For this review, take the finished solid that the model builds, in its own axes (mm). Round coordinates to 2 decimals unless told otherwise and drop trailing zeros. Loops run counter-clockwise (first coordinate to the right, second up) from the corner with the lowest first, then second, coordinate; pieces in that order, holes last. Notation, with made-up numbers: (58.25, 20) -> (86.25, 20) arc R12 ccw to (86.25, 40) -> close; hole circle Ø1 at (57.25, 26.5). An arc over 180 degrees is marked (long way). One line per question, with ' | ' between items. Start each with the question number.
1. Draft analysis for pull direction Y (two halves, no side actions). For faces 1 (the face through (0, 23, -208)), 2 (the face through (3.131, -25.395, -190.081)), 3 (the face through (3.131, 25.395, -190.919)), state which applies: pulls with the +Y half, pulls with the -Y half, needs draft (parallel to the pull), parting line crosses it, or undercut.
2. Consider section A-A (y = 76.2). Write out the cut boundary in (x, z), and give its area (3 significant figures).
3. Consider section C-C (x = 3.75). Count the separate pieces of the cut face and the enclosed holes in it, and give its area (3 significant figures).
4. Wall thickness on line 1 along Z through (x, y) = (5.25, -68.5); line 2 along Z through (x, y) = (1, 20); line 3 along Y through (x, z) = (5.25, -114): over which ranges is each line inside the solid? List them lowest first.
5. Consider section B-B (z = -194). Write out the cut boundary in (x, y).
```python
from build123d import *

# Parameters (mm, degrees)
BOSS_EXTRUDE1_DEPTH = 6.35
SKETCH2_R           = 1.7272
SKETCH2_R_2         = 1.3890625
SKETCH2_R_3         = 1.984375
CUT_EXTRUDE1_DEPTH  = 7.35


with BuildPart() as part:
    # Sketch1 → Boss-Extrude1 (new body)
    with BuildSketch(Plane(origin=(0, 0, 0), x_dir=(0, 0, -1), z_dir=(1, 0, 0))):
        Polygon((146.05, 95.25), (158.75, 95.25), (552.45, 95.25), (552.45, -95.25), (158.75, -95.25), (146.05, -95.25), (-146.05, -95.25), (-146.05, 95.25), align=None)
    extrude(amount=BOSS_EXTRUDE1_DEPTH)

    # Sketch2 → Cut-Extrude1 (cut, through all)
    with BuildSketch(Plane.ZY):
        with Locations((113.660651072, 53.713174026)):
            Circle(SKETCH2_R)
        with Locations((75.560651072, 53.713174026)):
            Circle(SKETCH2_R)
        with Locations((37.460651072, 53.713174026)):
            Circle(SKETCH2_R)
        with Locations((-0.639348928, 53.713174026)):
            Circle(SKETCH2_R)
        with Locations((-38.739348928, 53.713174026)):
            Circle(SKETCH2_R)
        with Locations((-76.839348928, 53.713174026)):
            Circle(SKETCH2_R)
        with Locations((-114.939348928, 53.713174026)):
            Circle(SKETCH2_R)
        with Locations((-114.939348928, 2.913174026)):
            Circle(SKETCH2_R)
        with Locations((-76.839348928, 2.913174026)):
            Circle(SKETCH2_R)
        with Locations((-38.739348928, 2.913174026)):
            Circle(SKETCH2_R)
        with Locations((-0.639348928, 2.913174026)):
            Circle(SKETCH2_R)
        with Locations((37.460651072, 2.913174026)):
            Circle(SKETCH2_R)
        with Locations((75.560651072, 2.913174026)):
            Circle(SKETCH2_R)
        with Locations((113.660651072, 2.913174026)):
            Circle(SKETCH2_R)
        with Locations((92.336825974, -67.314348928)):
            Circle(SKETCH2_R)
        with Locations((41.536825974, -67.314348928)):
            Circle(SKETCH2_R)
        with Locations((-47.363174026, -67.314348928)):
            Circle(SKETCH2_R)
        with Locations((-98.163174026, -67.314348928)):
            Circle(SKETCH2_R)
        with Locations((-227.452489037, 52.197)):
            Circle(SKETCH2_R)
        with Locations((-227.452489037, -52.197)):
            Circle(SKETCH2_R)
        with Locations((-409.722889037, -52.197)):
            Circle(SKETCH2_R)
        with Locations((-409.722889037, 52.197)):
            Circle(SKETCH2_R)
        with Locations((-522.859, -17.782353467)):
            Circle(SKETCH2_R_2)
        with Locations((-479.806, -17.78)):
            Circle(SKETCH2_R_2)
        with Locations((-479.806, -65.532)):
            Circle(SKETCH2_R_2)
        with Locations((-522.859, -65.532)):
            Circle(SKETCH2_R_2)
        with Locations((-462.026, 46.355)):
            Circle(SKETCH2_R_3)
        with Locations((-518.668, 19.685)):
            Circle(SKETCH2_R_3)
        with BuildLine():
            Line((-501.65, 82.55), (-476.25, 82.55))
            ThreePointArc((-476.25, 82.55), (-469.9, 76.2), (-476.25, 69.85))
            Line((-476.25, 69.85), (-501.65, 69.85))
            ThreePointArc((-501.65, 69.85), (-508, 76.2), (-501.65, 82.55))
        make_face()
        with BuildLine():
            Line((-171.45, 6.35), (-171.45, -6.35))
            ThreePointArc((-171.45, -6.35), (-190.5, -25.4), (-209.55, -6.35))
            Line((-209.55, -6.35), (-209.55, 6.35))
            ThreePointArc((-209.55, 6.35), (-190.5, 25.4), (-171.45, 6.35))
        make_face()
    extrude(amount=-CUT_EXTRUDE1_DEPTH, mode=Mode.SUBTRACT)


solid = part.part
```
Answer block:
1) face 1: needs draft | face 2: undercut | face 3: undercut
2) outline: (0, -552.45) -> (6.35, -552.45) -> (6.35, -508) -> (0, -508) -> close; (0, -469.9) -> (6.35, -469.9) -> (6.35, 146.05) -> (0, 146.05) -> close | area: 4,190 mm2
3) separate pieces: 1 | enclosed holes: 30 | area: 131,000 mm2
4) line 1: z = -552.45 to -99.42, -96.91 to -48.62, -46.11 to 40.28, 42.79 to 91.08, 93.59 to 146.05 | line 2: z = -552.45 to -520.63, -516.71 to -203.79, -177.21 to 146.05 | line 3: y = -95.25 to 1.46, 4.36 to 52.26, 55.16 to 95.25
5) outline: (0, -95.25) -> (6.35, -95.25) -> (6.35, -25.08) -> (0, -25.08) -> close; (0, 25.08) -> (6.35, 25.08) -> (6.35, 95.25) -> (0, 95.25) -> close
